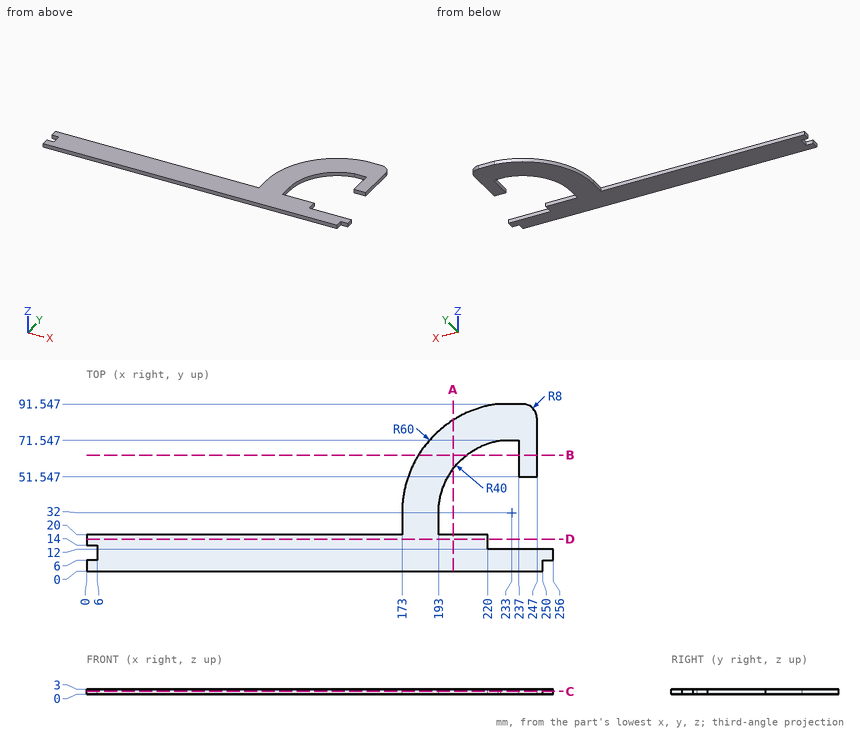
Geometry: see drawing. Coordinates: mm, zero at the bounding-box minimum. Round coordinates to 2 decimals unless told otherwise and drop trailing zeros. Loops run counter-clockwise (first coordinate to the right, second up) from the corner with the lowest first, then second, coordinate; pieces in that order, holes last. Notation, with made-up numbers: M -1,4.5 L 30,4.5 A12 cw 30,26.5 Z; hole C -2,64 d10. An arc over 180 degrees is marked long. Use a Markdown table: item, result. Add a question column.
1. Ray query, line 1 along X through (y, z) = (34, 2.1); line 2 along Y through (x, z) = (32, 0.75); line 3 along X through (y, z) = (61.5, 0.3) (1 decimal). Return the intervals inside material, ascending. Write a range as [from, to].
2. Cut plane B-B, the plane y = 63.5. Output: boundary loops of the cut face in (x, z).
3. Cut plane D-D, the plane y = 17.5. Output: boundary loops of the cut face in (x, z).
4. Contact query for flat-ended pins moving along their axis: pin 1 (1.5 mm diameter, centred on x = 201.5, z = 1.5, fed in from +Y); pin 2 (0.9 mm diameter, centred on y = 18, z = 1.5, fed in from +X); pin 3 (1.5 mm diameter, centred on x = 253.5, z = 1.5, fed in from -Y); pin 4 (5 mm diameter, centred on x = 55.5, y = 20.5, fed in from -Z). Output: stop coordinate, or through.
5. Cut plane A-A, the plane x = 201. Output: boundary loops of the cut face in (y, z) (1 decimal), and give its area (3 significant figures).
6. Cut plane C-C, the plane z = 1.7. Output: boundary loops of the cut face in (x, y) (1 decimal).
Solution:
| question | item | result |
|---|---|---|
| 1 | line 1 | x = [173.03, 193.05] |
| 1 | line 2 | y = [0, 20] |
| 1 | line 3 | x = [180.8, 206], [237, 247] |
| 2 | outline | M 181.93,0 L 208.35,0 L 208.35,3 L 181.93,3 Z; M 237,0 L 247,0 L 247,3 L 237,3 Z |
| 3 | outline | M 0,0 L 220,0 L 220,3 L 0,3 Z |
| 4 | pin 1 | stops at y = 83.52 |
| 4 | pin 2 | stops at x = 220 |
| 4 | pin 3 | stops at y = 6 |
| 4 | pin 4 | stops at z = 0 |
| 5 | outline | M 0,0 L 20,0 L 20,3 L 0,3 Z; M 56,0 L 82.8,0 L 82.8,3 L 56,3 Z |
| 5 | area | 140 mm2 |
| 6 | outline | M 0,0 L 250,0 L 250,6 L 256,6 L 256,12 L 220,12 L 220,20 L 193,20 L 193,32 A40 cw 227,71.5 L 237,71.5 L 237,51.5 L 247,51.5 L 247,83.5 A8 ccw 239,91.5 L 225.6,91.5 A60 ccw 173,32 L 173,20 L 0,20 L 0,14 L 6,14 L 6,6 L 0,6 Z |
